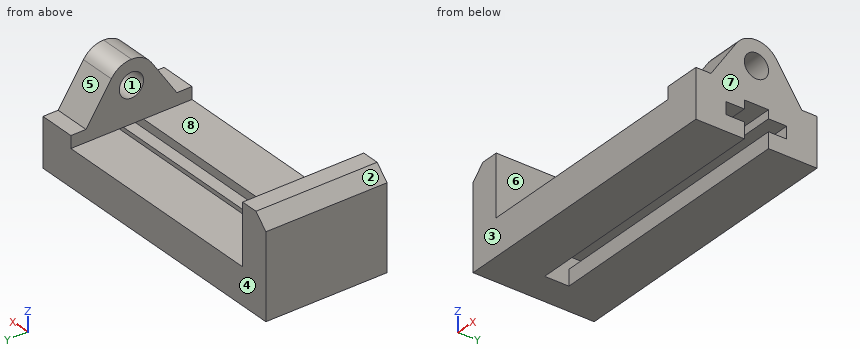
```python
from build123d import *

# Parameters (mm, degrees)
F1_DEPTH = 127
F3_DEPTH = 273.05
F4_R     = 12.7
F5_DEPTH = 50.8
F6_DEPTH = 50.8


with BuildPart() as f1:
    # F0 (on Front) → F1 (new body)
    with BuildSketch(Plane.XZ):
        Polygon((0, 88.129619), (0, 0), (304.8, 0), (304.8, 101.600003), (266.7, 101.600003), (266.7, 38.1), (31.75, 38.1), (31.75, 101.600003), (13.470384, 101.600003), align=None)
    extrude(amount=-F1_DEPTH)

    # F2 (on face) → F3 (cut)
    with BuildSketch(Plane.YZ.offset(304.8)):
        Polygon((50.8, 16.51), (50.8, 0), (76.2, 0), (76.2, 16.51), (95.25, 16.51), (95.25, 29.21), (76.2, 29.21), (76.2, 38.1), (50.8, 38.1), (50.8, 29.21), (31.75, 29.21), (31.75, 16.51), align=None)
    extrude(amount=-F3_DEPTH, mode=Mode.SUBTRACT)

    # F4 (on face) → F5 (cut)
    with BuildSketch(Plane.YZ.offset(304.8)):
        with Locations((63.5, 76.200003)):
            Circle(F4_R)
    extrude(amount=-F5_DEPTH, mode=Mode.SUBTRACT)

    # F4 (on face) → F6 (cut)
    with BuildSketch(Plane.YZ.offset(304.8)):
        with BuildLine():
            Line((0, 101.600003), (0, 50.8))
            Line((0, 50.8), (15.875, 50.8))
            Line((15.875, 50.8), (42.406574, 90.350175))
            ThreePointArc((42.406574, 90.350175), (51.547058, 98.611767), (63.5, 101.600003))
            Line((63.5, 101.600003), (0, 101.600003))
        make_face()
        with BuildLine():
            Line((127, 101.600003), (63.5, 101.600003))
            ThreePointArc((63.5, 101.600003), (75.452942, 98.611767), (84.593426, 90.350175))
            Line((84.593426, 90.350175), (111.125, 50.8))
            Line((111.125, 50.8), (127, 50.8))
            Line((127, 50.8), (127, 101.600003))
        make_face()
    extrude(amount=-F6_DEPTH, mode=Mode.SUBTRACT)


solid = f1.part
```
Build history of the part. All positions in model axes, mm. Face numbers are marked on the shaded views. A direction names the side the tool comes from. Round coordinates to 2 decimals unless told otherwise and drop trailing zeros. Loops run counter-clockwise (first coordinate to the right, second up) from the corner with the lowest first, then second, coordinate; pieces in that order, holes last.
Item 1: Saw through at C-C (y = 59). List the corners of the cut face in (x, z).
Item 2: Drill centre lines: line 1 along Y through (x, z) = (176, 22); line 2 along X through (y, z) = (85, 84); line 3 along Z through (x, y) = (293, 63). Where is each one in solid material? Low to high.
Item 3: Pin check, flat tips, straight feed: P1, Ø14, axis at x = 144, z = 21, coming from the -Y side; P2, Ø9.5, axis at x = 181.5, y = 40, coming from the +Z side; P3, Ø17.5, axis at x = 281, y = 10, coming from the +Z side; P4, Ø7.5, axis at x = 276.5, y = 60.5, coming from the -Z side. Stop position of each tip, or through.
Item 4: Saw through at D-D (z = 24.5). List the corners of the cut face in (x, y).
Item 5: Two-plate mould, pull along Y, no slides. Class the marked faces 1, 2, 3 and 4: released by +Y, released by -Y, zero draft, split by the parting line, or undercut.
Item 6: Saw through at A-A (x = 94). List the corners of the cut face in (y, z).
Item 7: Saw through at B-B (z = 56). List the corners of the cut face in (x, y).
Item 8: Which spindle directions (+Z, -Z, +X, -X, +Y, -Y) get a long thin tool onto all of the face, cutting with end or side? Do the marked faces 5, 6, 7 and 8. Say none if no direction does.
Worked answers:
1. outline: (0, 0) - (31.75, 0) - (31.75, 101.6) - (13.47, 101.6) - (0, 88.13) - close; (266.7, 38.1) - (304.8, 38.1) - (304.8, 64.32) - (266.7, 64.32) - close; (266.7, 88.08) - (304.8, 88.08) - (304.8, 101.2) - (266.7, 101.2) - close
2. line 1: y = 0 to 31.75, 95.25 to 127
2. line 2: x = 0 to 31.75, 266.7 to 304.8
2. line 3: z = 38.1 to 63.51, 88.89 to 101.6
3. P1: stops at y = 0
3. P2: stops at z = 38.1
3. P3: stops at z = 55.09
3. P4: stops at z = 38.1
4. outline: (0, 0) - (304.8, 0) - (304.8, 31.75) - (31.75, 31.75) - (31.75, 95.25) - (304.8, 95.25) - (304.8, 127) - (0, 127) - close
5. face 1: undercut
5. face 2: zero draft
5. face 3: released by -Y
5. face 4: released by +Y
6. outline: (0, 0) - (50.8, 0) - (50.8, 16.51) - (31.75, 16.51) - (31.75, 29.21) - (50.8, 29.21) - (50.8, 38.1) - (0, 38.1) - close; (76.2, 0) - (127, 0) - (127, 38.1) - (76.2, 38.1) - (76.2, 29.21) - (95.25, 29.21) - (95.25, 16.51) - (76.2, 16.51) - close
7. outline: (0, 0) - (31.75, 0) - (31.75, 127) - (0, 127) - close; (266.7, 19.36) - (304.8, 19.36) - (304.8, 107.64) - (266.7, 107.64) - close
8. face 5: +Z, +X, +Y
8. face 6: none
8. face 7: +Z, -Z, +X, +Y, -Y
8. face 8: +Z, +Y, -Y
